For this review, use the dimensioned drawing (mm, ordinates from the lowest corner) and the shaded views. Coordinates: 2 decimals unless noted, no trailing zeros. One line per item, written item: value.
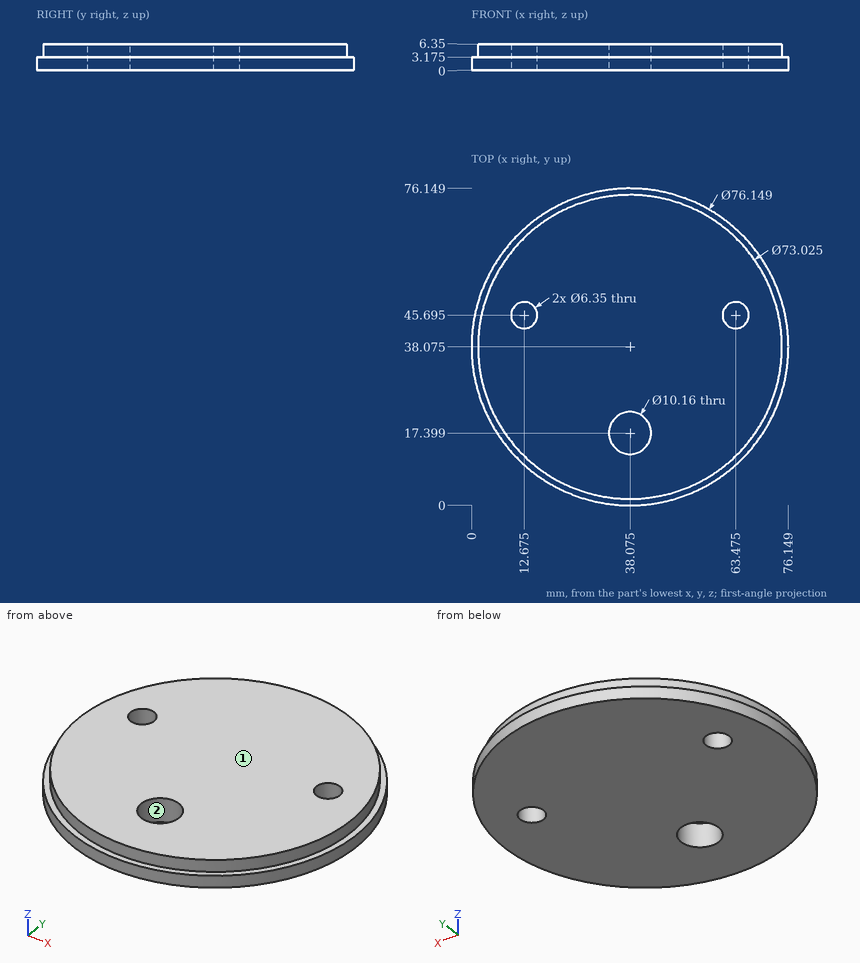
(1) Mouldability with a two-part tool opening along Y and no side actions: class the marked faces 1 and 2 as released by +Y, released by -Y, zero draft, split by the parting line, or undercut.
Reply:
face 1: zero draft
face 2: undercut
(2) Insertion check: pin 1 (2 mm diameter, centred on x = 55, z = 3.5, fed in from +Y); pin 2 (1.5 mm diameter, centred on x = 27, z = 4, fed in from -Y); pin 3 (1.5 mm diameter, centred on y = 64, z = 1.5, fed in from +X). Each pin has a flat end and moves straight along its axis. Give the tip position at first contact, or say it passes through.
Reply:
pin 1: stops at y = 72.63
pin 2: stops at y = 3.05
pin 3: stops at x = 66.64
(3) To check wall thickness, follow line 1 along X through (y, z) = (38, 5); line 2 along Y through (x, z) = (34, 3.5) (1 decimal); line 3 along X through (y, z) = (61, 3.25) (1 decimal). State the ranges of each line that lie inside material, in increasing order. Write a range as [from, to].
Reply:
line 1: x = [1.56, 74.59]
line 2: y = [1.8, 14.4], [20.4, 74.4]
line 3: x = [9.7, 66.5]
